Design review of the part built by this model. Coordinates are the model's own, in mm. Face numbers are marked on the shaded views. A direction names the side the tool comes from. Give positions to 0.01 mm unless a question says otherwise; leave off trailing zeros. Write each loop counter-clockwise with the first axis right and the second up, starting at its lowest first coordinate (ties: lowest second). Pieces come first, ordered by that corner, then holes. Notation, with made-up numbers: M 85,77.25 L 130,77.25 A7 ccw 130,89.25 Z; hole C -6.75,68.5 d11. An arc over 180 degrees is marked long. Use one line per item in the form item = value. Start each with the question number.
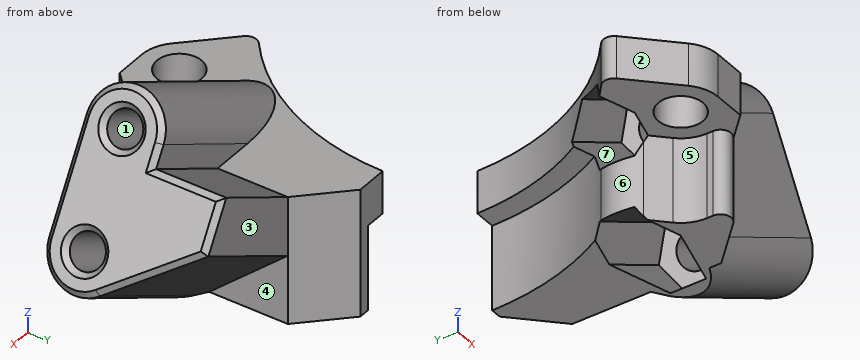
from build123d import *

# Parameters (mm, degrees)
SKETCH1_R           = 2.100000000000001
BOSS_EXTRUDE1_DEPTH = 12
BOSS_EXTRUDE2_START = -6.21
BOSS_EXTRUDE2_DEPTH = 13.79
CUT_EXTRUDE1_DEPTH  = 8
BOSS_EXTRUDE3_REACH = 41.051
SKETCH4_R           = 1.6
SKETCH4_R_2         = 1.6000000000000019
CUT_EXTRUDE2_DEPTH  = 40.05068839257359
CHAMFER2_SIZE       = 4
CUT_EXTRUDE3_REACH  = 41.051
CHAMFER3_SIZE       = 6
CUT_EXTRUDE4_START  = -12.5
CUT_EXTRUDE4_DEPTH  = 27.550688504002913
FILLET1_R           = 1
CHAMFER4_SIZE       = 0.5
FILLET2_R           = 3


with BuildPart() as part:
    # Sketch1 → Boss-Extrude1 (new body)
    with BuildSketch(Plane.XY):
        with BuildLine():
            Line((13.241359911348773, -18.191107379654646), (18.031222920256923, -22.980970388562806))
            ThreePointArc((18.031222920256923, -22.980970388562806), (19.166704641132032, -23.73967501819941), (20.50609665440986, -24.006096654409898))
            Line((20.50609665440986, -24.006096654409898), (29.499999999999993, -24.006096654409898))
            Line((29.499999999999993, -24.006096654409898), (29.499999999999993, 3.7e-16))
            Line((29.499999999999993, 3.7e-16), (22.500000000000007, 1.32e-15))
            ThreePointArc((22.500000000000007, 1.32e-15), (20.052189381777588, -10.205866009179541), (13.241359911348773, -18.191107379654646))
        make_face()
        with Locations((20.506096654409866, -20.5060966544099)):
            Circle(SKETCH1_R, mode=Mode.SUBTRACT)
    extrude(amount=BOSS_EXTRUDE1_DEPTH)

    # Sketch2 → Boss-Extrude2 (add)
    with BuildSketch(Plane.XZ.offset(24.006096654409898).offset(BOSS_EXTRUDE2_START)):
        Polygon((36.42820323027541, 1.1e-16), (29.499999999999993, 0), (29.499999999999993, 12), (38.1602540378444, 16.99999999999995), (45.08845726811982, 4.999999999999951), align=None)
    extrude(amount=-BOSS_EXTRUDE2_DEPTH)

    # Sketch3 → Cut-Extrude1 (cut)
    with BuildSketch(Plane(origin=(0, 0, 0), x_dir=(-1, 0, 0), z_dir=(0, 0, -1))):
        with BuildLine():
            Line((-18.031222920256923, -22.980970388562806), (-14.671554465329313, -19.621301933635188))
            ThreePointArc((-14.671554465329313, -19.621301933635188), (17.324116139070405, 17.324116139070437), (-19.621301933635156, -14.671554465329354))
            Line((-19.621301933635156, -14.671554465329354), (-22.98097038856278, -18.031222920256983))
            ThreePointArc((-22.98097038856278, -18.031222920256983), (-23.739675018199375, -19.1667046411321), (-24.00609665440987, -20.506096654409927))
            Line((-24.00609665440987, -20.506096654409927), (-24.00609665440987, -24.0060966544099))
            Line((-24.00609665440987, -24.0060966544099), (-20.50609665440986, -24.006096654409905))
            ThreePointArc((-20.50609665440986, -24.006096654409905), (-19.166704641132036, -23.739675018199403), (-18.031222920256923, -22.980970388562806))
        make_face()
    extrude(amount=-CUT_EXTRUDE1_DEPTH, mode=Mode.SUBTRACT)

    # Boss-Extrude3: up to this plane
    boss_extrude3_end = Plane(origin=(0, 0, 12), z_dir=(0, 0, 1))
    # Sketch5 → Boss-Extrude3 (add, up to the surface)
    with BuildSketch(Plane(origin=(35.98140646055117, 0, 20.77387470582027), x_dir=(0.4999999999999946, 0, -0.8660254037844417), z_dir=(0.8660254037844417, 0, 0.4999999999999946)), mode=Mode.PRIVATE) as boss_extrude3_sk1:
        with BuildLine():
            Line((2.357695154586543, -10.5960966544099), (4.357695154586543, -10.5960966544099))
            Line((4.357695154586543, -10.5960966544099), (4.357695154586545, -17.796096654409897))
            Line((4.357695154586545, -17.796096654409897), (2.3576951545865437, -17.796096654409897))
            ThreePointArc((2.3576951545865437, -17.796096654409897), (-1.2423048454134564, -14.1960966544099), (2.357695154586543, -10.5960966544099))
        make_face()
    boss_extrude3_tool1 = split(extrude(boss_extrude3_sk1.sketch, amount=-BOSS_EXTRUDE3_REACH, mode=Mode.PRIVATE), bisect_by=boss_extrude3_end, keep=Keep.BOTH, mode=Mode.PRIVATE)
    add(boss_extrude3_tool1.solids().sort_by_distance((36.919961, -14.196097, 19.148251))[0])

    # Sketch4 → Cut-Extrude2 (cut, through all)
    with BuildSketch(Plane(origin=(35.98140646055118, 0, 20.773874705820273), x_dir=(0.49999999999999495, 0, -0.8660254037844417), z_dir=(0.8660254037844417, 0, 0.49999999999999495))):
        with Locations((2.357695154586536, -14.2)):
            Circle(SKETCH4_R)
        with Locations((12.357695154586537, -14.2)):
            Circle(SKETCH4_R_2)
    extrude(amount=-CUT_EXTRUDE2_DEPTH, mode=Mode.SUBTRACT)

    # Chamfer2
    chamfer2_edges = [part.edges().sort_by_distance(p)[0] for p in [
        (29.499999999999993, 3.7e-16, 6),
    ]]
    chamfer(chamfer2_edges, length=CHAMFER2_SIZE)

    # Cut-Extrude3: up to this plane
    cut_extrude3_end = Plane(origin=(29.499999999999993, -24.006096654409898, 12), z_dir=(-1, 0, 0))
    # Sketch7 → Cut-Extrude3 (cut, up to the surface)
    with BuildSketch(Plane(origin=(35.98140646055117, 0, 20.77387470582027), x_dir=(0.4999999999999946, 0, -0.8660254037844417), z_dir=(0.8660254037844417, 0, 0.4999999999999946)), mode=Mode.PRIVATE) as cut_extrude3_sk1:
        with BuildLine():
            Line((15.22937626137959, -12.028952413951306), (9.16393898536506, -4.0060966544099))
            Line((9.16393898536506, -4.0060966544099), (22.041886428240783, -4.0060966544099))
            Line((22.041886428240783, -4.0060966544099), (22.041886428240783, -24.0060966544099))
            Line((22.041886428240783, -24.0060966544099), (2.357695154586543, -24.006096654409905))
            Line((2.357695154586543, -24.006096654409905), (2.357695154586542, -17.796096654409897))
            Line((2.357695154586542, -17.796096654409897), (12.357695154586544, -17.8))
            ThreePointArc((12.357695154586544, -17.8), (15.580719457145811, -15.803781264734175), (15.22937626137959, -12.028952413951306))
        make_face()
    cut_extrude3_tool1 = split(extrude(cut_extrude3_sk1.sketch, amount=-CUT_EXTRUDE3_REACH, mode=Mode.PRIVATE), bisect_by=cut_extrude3_end, keep=Keep.BOTH, mode=Mode.PRIVATE)
    add(cut_extrude3_tool1.solids().sort_by_distance((42.191658, -7.848292, 10.017403))[0], mode=Mode.SUBTRACT)

    # Chamfer3
    chamfer3_edges = [part.edges().sort_by_distance(p)[0] for p in [
        (29.499999999999993, -24.006096654409898, 6),
    ]]
    chamfer(chamfer3_edges, length=CHAMFER3_SIZE)

    # Sketch8 → Cut-Extrude4 (cut, through all)
    with BuildSketch(Plane(origin=(35.98140646055117, 0, 20.77387470582027), x_dir=(0.4999999999999946, 0, -0.8660254037844417), z_dir=(0.8660254037844417, 0, 0.4999999999999946)).offset(CUT_EXTRUDE4_START)):
        Polygon((5.257695154586542, -15.874315780649912), (5.257695154586541, -12.525684219350083), (2.3576951545865397, -10.85136843870017), (-0.5423048454134567, -12.525684219350083), (-0.5423048454134562, -15.874315780649912), (2.3576951545865446, -17.54863156129983), align=None)
        Polygon((9.457695154586544, -12.525684219350088), (9.457695154586544, -15.874315780649908), (12.35769515458654, -17.54863156129982), (15.257695154586537, -15.874315780649905), (15.257695154586537, -12.525684219350087), (12.357695154586539, -10.851368438700176), align=None)
    extrude(amount=-CUT_EXTRUDE4_DEPTH, mode=Mode.SUBTRACT)

    # Fillet1
    fillet1_edges = [part.edges().sort_by_distance(p)[0] for p in [
        (13.241359911348777, -18.191107379654646, 10),
        (24.00609665440987, -23.50000000000002, 4),
    ]]
    fillet(fillet1_edges, radius=FILLET1_R)

    # Chamfer4
    chamfer4_edges = [part.edges().sort_by_distance(p)[0] for p in [
        (36.36025403784444, -14.2, 20.11769145362395),
        (41.36025403784439, -14.2, 11.457437415779536),
        (39.70215336073716, -17.796096654409897, 14.329352032593636),
        (35.36025403784445, -14.1960966544099, 21.849742261192826),
        (37.660254037844425, -10.5960966544099, 17.866025403784395),
        (38.1602540378444, -7.3010966544099, 16.99999999999995),
        (39.36181499553902, -4.006096654409898, 14.918835372881723),
        (42.079735272237265, -8.017524534180602, 10.211259362718662),
        (43.790000296334796, -15.728302500078335, 7.2489934465736905),
    ]]
    chamfer(chamfer4_edges, length=CHAMFER4_SIZE)

    # Fillet2
    fillet2_edges = [part.edges().sort_by_distance(p)[0] for p in [
        (19.621301933635156, -14.671554465329354, 2.8324293970035703),
    ]]
    fillet(fillet2_edges, radius=FILLET2_R)


solid = part.part
1. Clearance check with flat-ended pins moving along their axes: pin 1 Ø5 at (x, y) = (19.5, -7.5) entering from +Z; pin 2 Ø3 at (x, z) = (34.5, 14) entering from +Y; pin 3 Ø6 at (x, y) = (18, -20) entering from -Z. State where each tip first meets the part, or that it passes through.
2. We need section B-B (x = 17). State the section outline as (y, z) points.
3. To check wall thickness, follow L1, parallel to Y at x = 34, z = 16.75; L2, parallel to Z at x = 16.75, y = -20; L3, parallel to Z at x = 31.25, y = -14. State the ranges of each line that lie inside material, in increasing order.
4. We need section A-A (y = -6.5). State the section outline as (x, z) points, and give its area (3 significant figures).
5. For the marked faces 4, 5, 6 and 7, list the 3-axis set-ups (+Z, -Z, +X, -X, +Y, -Y) from which the entire face can be reached by the end or side of a thin tool; tool diameter is ignored.
6. We need section C-C (y = -14.75). Give the number of separate pieces and of enclosed holes in the cut face, and give its area (3 significant figures).
7. Draft analysis for pull direction X (two halves, no side actions). For the marked faces 1, 2 and 3, state which applies: pulls with the +X half, pulls with the -X half, needs draft (parallel to the pull), parting line crosses it, or undercut.
Answer block:
q1.pin_1 = 12
q1.pin_2 = -4.01
q1.pin_3 = 8
q2.outline = M -21.95,8 L -17.09,8 L -15.87,10.44 L -14.74,10.44 L -14.74,12 L -21.95,12 Z
q3.L1 = -17.8 to -15.79, -12.61 to -10.6
q3.L2 = 8 to 12
q3.L3 = 0 to 0.42, 5.61 to 13.49, 17.15 to 19.47
q4.outline = M 21.54,8 L 23.62,8 L 23.62,0 L 29.5,0 L 29.5,4.27 L 41.07,10.95 L 41.19,11.75 L 38.41,16.57 L 37.73,16.75 L 29.5,12 L 21.54,12 Z
q4.area = 158 mm^2
q5.face_4 = -Z, +X, +Y
q5.face_5 = -Z, -X, -Y
q5.face_6 = -Z, -X
q5.face_7 = none
q6.separate_pieces = 3
q6.enclosed_holes = 0
q6.area = 186 mm^2
q7.face_1 = undercut
q7.face_2 = pulls with the -X half
q7.face_3 = needs draft
